For this review, take the finished solid that the model builds, in its own axes (mm). Round coordinates to 2 decimals unless told otherwise and drop trailing zeros. Loops run counter-clockwise (first coordinate to the right, second up) from the corner with the lowest first, then second, coordinate; pieces in that order, holes last.
1. Consider section A-A on y = -3.75. State the section outline as (x, z) points, then the cut area to 3 significant figures.
2. Consider section B-B on z = -3. State the section outline as (x, y) points.
3. To check wall thickness, follow line 1 along Y through (x, z) = (0.1, 1); line 2 along Z through (x, y) = (0.1, 5); line 3 along Y through (x, z) = (0, 0). State the ranges of each line that lie inside material, in increasing order.
4. Consider section C-C on z = 1. State the section outline as (x, y) points, then the cut area to 3 significant figures.
5. Consider section D-D on y = 5.25. State the section outline as (x, z) points.
from build123d import *

# Parameters (mm, degrees)
SKETCH3_R                = 0.5207
BOSS_EXTRUDE1_DEPTH      = 0.3175
BOSS_EXTRUDE1_DEPTH_BACK = 0.3175
FILLET1_R                = 0.7874


with BuildPart() as part:
    # Sketch3 → Boss-Extrude1 (new body, two sides)
    with BuildSketch(Plane(origin=(0, 0, 0), x_dir=(0, 0, -1), z_dir=(1, 0, 0))) as boss_extrude1_sk:
        with BuildLine():
            Line((-1.790070495, 6.49754857), (-2.532309488, 4.3891842))
            ThreePointArc((-2.532309488, 4.3891842), (0, -5.5626), (2.532309488, 4.3891842))
            Line((2.532309488, 4.3891842), (1.790070495, 6.49754857))
            Line((1.790070495, 6.49754857), (0.113925819, 6.526805784))
            Line((0.113925819, 6.526805784), (0.0749162, 4.291946216))
            ThreePointArc((0.0749162, 4.291946216), (0, -4.2926), (-0.0749162, 4.291946216))
            Line((-0.0749162, 4.291946216), (-0.113925819, 6.526805784))
            Line((-0.113925819, 6.526805784), (-1.790070495, 6.49754857))
        make_face()
        with Locations((-0.932493347, 5.394747393)):
            Circle(SKETCH3_R, mode=Mode.SUBTRACT)
        with Locations((0.932493347, 5.394747393)):
            Circle(SKETCH3_R, mode=Mode.SUBTRACT)
    extrude(amount=BOSS_EXTRUDE1_DEPTH)
    extrude(boss_extrude1_sk.sketch, amount=-BOSS_EXTRUDE1_DEPTH_BACK)

    # Fillet1
    fillet1_edges = [part.edges().sort_by_distance(p)[0] for p in [
        (0, 4.3891842, 2.532309488),
        (0, 6.49754857, 1.790070495),
        (0, 4.291946216, 0.0749162),
        (0, 4.291946216, -0.0749162),
        (0, 6.49754857, -1.790070495),
        (0, 4.3891842, -2.532309488),
    ]]
    fillet(fillet1_edges, radius=FILLET1_R)


solid = part.part
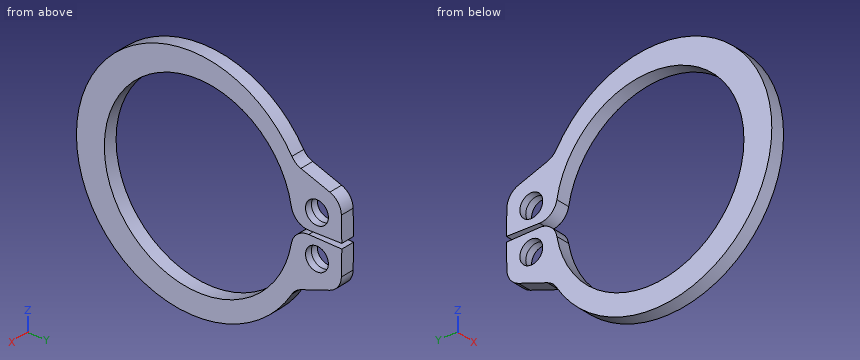
Resolved:
1. outline: (-0.32, -3.99) - (0.32, -3.99) - (0.32, -2.09) - (-0.32, -2.09) - close; (-0.32, 2.09) - (0.32, 2.09) - (0.32, 3.99) - (-0.32, 3.99) - close
1. area: 2.41 mm2
2. outline: (-0.32, -4.63) - (0.32, -4.63) - (0.32, -3.07) - (-0.32, -3.07) - close; (-0.32, 3.07) - (0.32, 3.07) - (0.32, 4.1) - (-0.32, 4.1) - close
3. line 1: y = -5.47 to -4.17, 4.17 to 4.88, 5.91 to 6.51
3. line 2: z = -2.32 to -1.27, -0.59 to -0.09, 0.09 to 0.59, 1.27 to 2.32
3. line 3: y = -5.56 to -4.29
4. outline: (-0.32, -5.47) - (0.32, -5.47) - (0.32, -4.17) - (-0.32, -4.17) - close; (-0.32, 4.17) - (0.32, 4.17) - (0.32, 4.88) - (-0.32, 4.88) - close; (-0.32, 5.91) - (0.32, 5.91) - (0.32, 6.51) - (-0.32, 6.51) - close
4. area: 1.65 mm2
5. outline: (-0.32, -2.23) - (0.32, -2.23) - (0.32, -1.43) - (-0.32, -1.43) - close; (-0.32, -0.43) - (0.32, -0.43) - (0.32, -0.09) - (-0.32, -0.09) - close; (-0.32, 0.09) - (0.32, 0.09) - (0.32, 0.43) - (-0.32, 0.43) - close; (-0.32, 1.43) - (0.32, 1.43) - (0.32, 2.23) - (-0.32, 2.23) - close
